Work out the finished part from the listing and answer in its coordinate system (mm). A direction names the side the tool comes from. Give positions to 0.01 mm unless a question says otherwise; leave off trailing zeros. Write each loop counter-clockwise with the first axis right and the second up, starting at its lowest first coordinate (ties: lowest second). Pieces come first, ordered by that corner, then holes.
1) Find section B-B (z = 2.1). Count the separate pieces of the cut face and the enclosed holes in it, plus the area to 3 significant figures.
2) Straight lines are drawn through the part: probe 1 along Y at (x, z) = (18.5, 0.3); probe 2 along Y at (x, z) = (8.5, 2.75); probe 3 along X at (y, z) = (22, 0.85). For each, find the intervals that lie inside material, in ascending order.
3) A tool of negligible diameter and unlimited length cuts with its end or side. For faces 5 (the face through (-39, 47.024, 1)), 6 (the face through (47.011, 0, 1)), 7 (the face through (-49, -9.976, 1)), from which of +Z, -Z, +X, -X, +Y, -Y can it reach the whole face along a straight path? Write none if from no direction.
4) Determine the mould class of faces 1 (the face through (10.011, -48, 1)), 2 (the face through (48, -9.976, 1)), 3 (the face through (-9.989, -48, 1)), 4 (the face through (-39.841, -39.983, 1.479)) for opening direction X: pulls with the +X half, pulls with the -X half, needs draft (parallel to the pull), parting line crosses it, or undercut.
5) Given pin 1 Ø1.5 at (x, z) = (-49, 1.5) entering from +Y; pin 2 Ø1.5 at (x, z) = (48.5, 1.5) entering from -Y; pin 3 Ø2.5 at (x, y) = (0, 10) entering from +Z; pin 4 Ø0.9 at (y, z) = (49, 2) entering from +X, each flat-ended and moving along its own axis, determine where each tip first touches the part or whether it passes through.
6) Find section C-C (x = 38). Determine the outline of the cut face in (y, z).
7) Find section A-A (y = 32.5). Determine the outline of the cut face in (x, z).
```python
from build123d import *

# Parameters (mm, degrees)
SKETCH_1_R      = 1
SKETCH_1_R_2    = 4
EXTRUDE_1_DEPTH = 3


with BuildPart() as part:
    # 草图1 → 凸台-拉伸1 (new body)
    with BuildSketch(Plane.XY):
        with BuildLine():
            Line((-10, 47.024429381), (10, 47.024429381))
            Line((10, 47.024429381), (10, 50.024429381))
            Line((10, 50.024429381), (30, 50.024429381))
            Line((30, 50.024429381), (30, 47.024429381))
            Line((30, 47.024429381), (47, 47.024429381))
            Line((47, 47.024429381), (47, 30.024429381))
            Line((47, 30.024429381), (49.989371297, 30.024429381))
            Line((49.989371297, 30.024429381), (49.989371297, 10.024429381))
            Line((49.989371297, 10.024429381), (47.010628703, 10.024429381))
            Line((47.010628703, 10.024429381), (47.010628703, -9.975570619))
            Line((47.010628703, -9.975570619), (50.010629304, -9.975570619))
            Line((50.010629304, -9.975570619), (50.010629304, -29.975570018))
            Line((50.010629304, -29.975570018), (47.010629304, -29.975570018))
            Line((47.010629304, -29.975570018), (47.010629304, -46.975570018))
            Line((47.010629304, -46.975570018), (30.010628703, -46.975570018))
            Line((30.010628703, -46.975570018), (30.010628703, -49.975570619))
            Line((30.010628703, -49.975570619), (10.010628703, -49.975570619))
            Line((10.010628703, -49.975570619), (10.010628703, -46.975570619))
            Line((10.010628703, -46.975570619), (-9.989371297, -46.975570619))
            Line((-9.989371297, -46.975570619), (-9.989371297, -49.975570619))
            Line((-9.989371297, -49.975570619), (-29.989371297, -49.975570619))
            Line((-29.989371297, -49.975570619), (-29.989371297, -46.975570619))
            Line((-29.989371297, -46.975570619), (-36.989371297, -46.975570619))
            ThreePointArc((-36.989371297, -46.975570619), (-39.918303485, -39.904502807), (-46.989371297, -36.975570619))
            Line((-46.989371297, -36.975570619), (-46.989371297, -29.975570619))
            Line((-46.989371297, -29.975570619), (-49.989371297, -29.975570619))
            Line((-49.989371297, -29.975570619), (-49.989371297, -9.975570619))
            Line((-49.989371297, -9.975570619), (-47.010628703, -9.975570619))
            Line((-47.010628703, -9.975570619), (-47.010628703, 10.024429381))
            Line((-47.010628703, 10.024429381), (-49.989371297, 10.024429381))
            Line((-49.989371297, 10.024429381), (-49.989371297, 30.024429381))
            Line((-49.989371297, 30.024429381), (-47, 30.024429381))
            Line((-47, 30.024429381), (-47, 47.024429381))
            Line((-47, 47.024429381), (-30, 47.024429381))
            Line((-30, 47.024429381), (-30, 50.024429381))
            Line((-30, 50.024429381), (-10, 50.024429381))
            Line((-10, 50.024429381), (-10, 47.024429381))
        make_face()
        with Locations((10, 0)):
            Circle(SKETCH_1_R, mode=Mode.SUBTRACT)
        with Locations((20, 0)):
            Circle(SKETCH_1_R, mode=Mode.SUBTRACT)
        with Locations((30, 0)):
            Circle(SKETCH_1_R, mode=Mode.SUBTRACT)
        with Locations((18.477666771, -7.653285964)):
            Circle(SKETCH_1_R, mode=Mode.SUBTRACT)
        with Locations((27.716462096, -11.480120288)):
            Circle(SKETCH_1_R, mode=Mode.SUBTRACT)
        with Locations((14.142428517, -14.141428517)):
            Circle(SKETCH_1_R, mode=Mode.SUBTRACT)
        with Locations((21.213496329, -21.212496329)):
            Circle(SKETCH_1_R, mode=Mode.SUBTRACT)
        with Locations((7.654285964, -18.476666771)):
            Circle(SKETCH_1_R, mode=Mode.SUBTRACT)
        with Locations((11.481120288, -27.715462096)):
            Circle(SKETCH_1_R, mode=Mode.SUBTRACT)
        with Locations((0.001, -19.999)):
            Circle(SKETCH_1_R, mode=Mode.SUBTRACT)
        with Locations((0.001, -29.999)):
            Circle(SKETCH_1_R, mode=Mode.SUBTRACT)
        with Locations((-7.652285964, -18.476666771)):
            Circle(SKETCH_1_R, mode=Mode.SUBTRACT)
        with Locations((-11.479120288, -27.715462096)):
            Circle(SKETCH_1_R, mode=Mode.SUBTRACT)
        with Locations((-14.140428517, -14.141428517)):
            Circle(SKETCH_1_R, mode=Mode.SUBTRACT)
        with Locations((-21.211496329, -21.212496329)):
            Circle(SKETCH_1_R, mode=Mode.SUBTRACT)
        with Locations((-18.475666771, -7.653285964)):
            Circle(SKETCH_1_R, mode=Mode.SUBTRACT)
        with Locations((-27.714462096, -11.480120288)):
            Circle(SKETCH_1_R, mode=Mode.SUBTRACT)
        with Locations((-19.998, 0)):
            Circle(SKETCH_1_R, mode=Mode.SUBTRACT)
        with Locations((-29.998, 0)):
            Circle(SKETCH_1_R, mode=Mode.SUBTRACT)
        with Locations((-18.475666771, 7.653285964)):
            Circle(SKETCH_1_R, mode=Mode.SUBTRACT)
        with Locations((-27.714462096, 11.480120288)):
            Circle(SKETCH_1_R, mode=Mode.SUBTRACT)
        with Locations((-14.140428517, 14.141428517)):
            Circle(SKETCH_1_R, mode=Mode.SUBTRACT)
        with Locations((-21.211496329, 21.212496329)):
            Circle(SKETCH_1_R, mode=Mode.SUBTRACT)
        with Locations((-7.652285964, 18.476666771)):
            Circle(SKETCH_1_R, mode=Mode.SUBTRACT)
        with Locations((-11.479120288, 27.715462096)):
            Circle(SKETCH_1_R, mode=Mode.SUBTRACT)
        with Locations((0.001, 19.999)):
            Circle(SKETCH_1_R, mode=Mode.SUBTRACT)
        with Locations((0.001, 29.999)):
            Circle(SKETCH_1_R, mode=Mode.SUBTRACT)
        with Locations((7.654285964, 18.476666771)):
            Circle(SKETCH_1_R, mode=Mode.SUBTRACT)
        with Locations((11.481120288, 27.715462096)):
            Circle(SKETCH_1_R, mode=Mode.SUBTRACT)
        with Locations((14.142428517, 14.141428517)):
            Circle(SKETCH_1_R, mode=Mode.SUBTRACT)
        with Locations((21.213496329, 21.212496329)):
            Circle(SKETCH_1_R, mode=Mode.SUBTRACT)
        with Locations((18.477666771, 7.653285964)):
            Circle(SKETCH_1_R, mode=Mode.SUBTRACT)
        with Locations((27.716462096, 11.480120288)):
            Circle(SKETCH_1_R, mode=Mode.SUBTRACT)
        with Locations((8.660254038, -5)):
            Circle(SKETCH_1_R, mode=Mode.SUBTRACT)
        with Locations((5, -8.660254038)):
            Circle(SKETCH_1_R, mode=Mode.SUBTRACT)
        with Locations((0, -10)):
            Circle(SKETCH_1_R, mode=Mode.SUBTRACT)
        with Locations((-5, -8.660254038)):
            Circle(SKETCH_1_R, mode=Mode.SUBTRACT)
        with Locations((-8.660254038, -5)):
            Circle(SKETCH_1_R, mode=Mode.SUBTRACT)
        with Locations((-10, 0)):
            Circle(SKETCH_1_R, mode=Mode.SUBTRACT)
        with Locations((-8.660254038, 5)):
            Circle(SKETCH_1_R, mode=Mode.SUBTRACT)
        with Locations((-5, 8.660254038)):
            Circle(SKETCH_1_R, mode=Mode.SUBTRACT)
        with Locations((0, 10)):
            Circle(SKETCH_1_R, mode=Mode.SUBTRACT)
        with Locations((5, 8.660254038)):
            Circle(SKETCH_1_R, mode=Mode.SUBTRACT)
        with Locations((8.660254038, 5)):
            Circle(SKETCH_1_R, mode=Mode.SUBTRACT)
        Circle(SKETCH_1_R_2, mode=Mode.SUBTRACT)
    extrude(amount=EXTRUDE_1_DEPTH)


solid = part.part
```
Results:
1. separate pieces: 1
1. enclosed holes: 45
1. area: 9,050 mm2
2. probe 1: y = -49.98 to -8.65, -6.65 to 6.65, 8.65 to 50.02
2. probe 2: y = -46.98 to -19.01, -17.94 to -5.99, -4.01 to 4.01, 5.99 to 17.94, 19.01 to 47.02
2. probe 3: x = -49.99 to -21.83, -20.6 to 20.6, 21.83 to 49.99
3. face 5: +Z, -Z, -X, +Y
3. face 6: +Z, -Z, +X
3. face 7: +Z, -Z, -X
4. face 1: undercut
4. face 2: needs draft
4. face 3: undercut
4. face 4: pulls with the -X half
5. pin 1: stops at y = 30.02
5. pin 2: stops at y = -29.98
5. pin 3: stops at z = 3
5. pin 4: stops at x = 30
6. outline: (-46.98, 0) - (47.02, 0) - (47.02, 3) - (-46.98, 3) - close
7. outline: (-47, 0) - (47, 0) - (47, 3) - (-47, 3) - close
